Geometry: final body of the model. Coordinates: model frame, mm. A direction names the side the tool comes from. Coordinates: 2 decimals unless noted, no trailing zeros. Write each loop counter-clockwise with the first axis right and the second up, starting at its lowest first coordinate (ties: lowest second). Pieces come first, ordered by that corner, then holes. Notation, with made-up numbers: M -40,5.5 L -28,5.5 A29 cw -28,25.5 Z; hole C 31.25,-13.75 d11. An arc over 180 degrees is marked long. Write item = value, one per line. Start each with the question number.
Item 1: Section C-C on y = 1.5. Output: boundary loops of the cut face in (x, z), plus the area to 3 significant figures.
Item 2: Pull-direction query (Z, two-part tool) for faces 4 (the cylindrical face through (1.036, 1.493, -0.325)), 5 (the flat face through (-5, -1, 0)), 6 (the cylindrical face through (2.725, 0.493, 0.715)); classes: +Z half, -Z half, draft (parallel to the pull), parting line (faces both ways), or undercut.
Item 3: Ray query, L1, parallel to X at y = 0.4, z = 0; L2, parallel to X at y = 1.15, z = 0.6; L3, parallel to X at y = 1.05, z = -1.15. Return the intervals inside material, ascending. Write a range as [from, to].
Item 4: Reachability of faces 1 (the flat face through (8, 1, 0)), 2 (the flat face through (-7, 2, 0)), 3 (the flat face through (0, 1, 0)) from +Z, -Z, +X, -X, +Y, -Y: full face, straight path, thin tool, end or side. Return the list, or none.
Item 5: Section D-D on x = -2.5. Output: boundary loops of the cut face in (y, z).
Item 6: Section B-B on x = 0. Output: boundary loops of the cut face in (y, z).
Item 7: Section A-A on y = 0.6. Output: boundary loops of the cut face in (x, z), plus the area to 3 significant figures.
Item 8: First-contact query: pin 1 Ø3 at (x, z) = (7, -1) entering from -Y; pin 2 Ø2 at (x, z) = (-7.5, 0) entering from -Y; pin 3 Ø0.8 at (x, z) = (-2.5, 0) entering from -Y. Flat tips, straight axial feed; report the tip coordinate or a pass-through.
from build123d import *

# Parameters (mm, degrees)
SKETCH1_R             = 1.5
BOSS_EXTRUDE1_DEPTH   = 2
BOSS_EXTRUDE1_2_DEPTH = 2
BOSS_EXTRUDE1_3_DEPTH = 2
BOSS_EXTRUDE1_4_DEPTH = 2
SKETCH1_3_W           = 20
SKETCH1_3_H           = 5
BOSS_EXTRUDE2_DEPTH   = 1
SKETCH1_4_R           = 0.75
CUT_EXTRUDE1_DEPTH    = 1
SKETCH1_5_W           = 20
SKETCH1_5_H           = 5
SKETCH1_5_W_2         = 18
SKETCH1_5_H_2         = 3
SKETCH1_5_R           = 1
BOSS_EXTRUDE3_DEPTH   = 1


with BuildPart() as part:
    # Sketch1 → Boss-Extrude1 (new body)
    with BuildSketch(Plane(origin=(0, 0, 0), x_dir=(1, 0, 0), z_dir=(0, 1, 0))):
        with Locations(Location((-7.5, 0, 0), (0, 0, 270))):
            Circle(SKETCH1_R)
    extrude(amount=BOSS_EXTRUDE1_DEPTH)



with BuildPart() as body_2:
    # Sketch1 → Boss-Extrude1 2 (new body)
    with BuildSketch(Plane(origin=(0, 0, 0), x_dir=(1, 0, 0), z_dir=(0, 1, 0))):
        with Locations(Location((-2.5, 0, 0), (0, 0, 270))):
            Circle(SKETCH1_R)
    extrude(amount=BOSS_EXTRUDE1_2_DEPTH)


with BuildPart() as body_3:
    # Sketch1 → Boss-Extrude1 3 (new body)
    with BuildSketch(Plane(origin=(0, 0, 0), x_dir=(1, 0, 0), z_dir=(0, 1, 0))):
        with Locations(Location((2.5, 0, 0), (0, 0, 270))):
            Circle(SKETCH1_R)
    extrude(amount=BOSS_EXTRUDE1_3_DEPTH)


with BuildPart() as body_4:
    # Sketch1 → Boss-Extrude1 4 (new body)
    with BuildSketch(Plane(origin=(0, 0, 0), x_dir=(1, 0, 0), z_dir=(0, 1, 0))):
        with Locations(Location((7.5, 0, 0), (0, 0, 270))):
            Circle(SKETCH1_R)
    extrude(amount=BOSS_EXTRUDE1_4_DEPTH)


with BuildPart() as part_1:
    add(part.part)

    add(body_2.part)  # Boss-Extrude2 merges body 2

    add(body_3.part)  # Boss-Extrude2 merges body 3

    add(body_4.part)  # Boss-Extrude2 merges body 4
    # Sketch1_3 → Boss-Extrude2 (add)
    with BuildSketch(Plane(origin=(0, 0, 0), x_dir=(1, 0, 0), z_dir=(0, 1, 0))):
        Rectangle(SKETCH1_3_W, SKETCH1_3_H)
    extrude(amount=BOSS_EXTRUDE2_DEPTH)

    # Sketch1_4 → Cut-Extrude1 (cut)
    with BuildSketch(Plane(origin=(0, 0, 0), x_dir=(1, 0, 0), z_dir=(0, 1, 0))):
        with Locations(Location((-7.5, 0, 0), (0, 0, 270))):
            Circle(SKETCH1_4_R)
        with Locations(Location((-2.5, 0, 0), (0, 0, 270))):
            Circle(SKETCH1_4_R)
        with Locations(Location((2.5, 0, 0), (0, 0, 270))):
            Circle(SKETCH1_4_R)
        with Locations(Location((7.5, 0, 0), (0, 0, 270))):
            Circle(SKETCH1_4_R)
    extrude(amount=CUT_EXTRUDE1_DEPTH, mode=Mode.SUBTRACT)

    # Sketch1_5 → Boss-Extrude3 (add)
    with BuildSketch(Plane(origin=(0, 0, 0), x_dir=(1, 0, 0), z_dir=(0, 1, 0))):
        Rectangle(SKETCH1_5_W, SKETCH1_5_H)
        Rectangle(SKETCH1_5_W_2, SKETCH1_5_H_2, mode=Mode.SUBTRACT)
        with BuildLine():
            ThreePointArc((-4, 0), (-5, 1), (-6, 0))
            Line((-6, 0), (-4, 0))
        make_face()
        with BuildLine():
            Line((-4, 0), (-6, 0))
            ThreePointArc((-6, 0), (-5, -1), (-4, 0))
        make_face()
        with Locations(Location((0, 0, 0), (0, 0, 270))):
            Circle(SKETCH1_5_R)
        with Locations(Location((5, 0, 0), (0, 0, 270))):
            Circle(SKETCH1_5_R)
    extrude(amount=-BOSS_EXTRUDE3_DEPTH)


solid = part_1.part
Responses:
q1.outline = C -7.5,0 d3; C -2.5,0 d3; C 2.5,0 d3; C 7.5,0 d3
q1.area = 28.3 mm²
q2.face_4 = parting line
q2.face_5 = draft
q2.face_6 = undercut
q3.L1 = [-10, -8.25], [-6.75, -3.25], [-1.75, 1.75], [3.25, 6.75], [8.25, 10]
q3.L2 = [-8.87, -6.13], [-3.87, -1.13], [1.13, 3.87], [6.13, 8.87]
q3.L3 = [-8.46, -6.54], [-3.46, -1.54], [1.54, 3.46], [6.54, 8.46]
q4.face_1 = -Y
q4.face_2 = +Z, -Z, +X, -X, +Y
q4.face_3 = +Y
q5.outline = M -1,-2.5 L 1,-2.5 L 1,-1.5 L 2,-1.5 L 2,1.5 L 1,1.5 L 1,2.5 L -1,2.5 L -1,1.5 L 0,1.5 L 0,0.75 L 1,0.75 L 1,-0.75 L 0,-0.75 L 0,-1.5 L -1,-1.5 Z
q6.outline = M -1,-2.5 L 1,-2.5 L 1,2.5 L -1,2.5 L -1,1.5 L 0,1.5 L 0,1 L -1,1 L -1,-1 L 0,-1 L 0,-1.5 L -1,-1.5 Z
q7.outline = M -10,-2.5 L 10,-2.5 L 10,2.5 L -10,2.5 Z; hole C -7.5,0 d1.5; hole C -2.5,0 d1.5; hole C 2.5,0 d1.5; hole C 7.5,0 d1.5
q7.area = 92.9 mm²
q8.pin_1 = -1
q8.pin_2 = 0
q8.pin_3 = 1
